```python
from build123d import *

# Parameters (mm, degrees)
SKETCH_1_R          = 1.5
EXTRUDE_1_DEPTH     = 3
SKETCH_2_R          = 1.5
EXTRUDE_4_DEPTH     = 6
FILLET_1_R          = 1
SKETCH_3_R          = 1.5
CUT_EXTRUDE_1_DEPTH = 10


with BuildPart() as part:
    # ｽｹｯﾁ1 → ﾎﾞｽ - 押し出し1 (new body)
    with BuildSketch(Plane.XY):
        with BuildLine():
            Line((-3, 0), (-3, -30))
            ThreePointArc((-3, -30), (0, -33), (3, -30))
            Line((3, -30), (3, 0))
            ThreePointArc((3, 0), (0, 3), (-3, 0))
        make_face()
        Circle(SKETCH_1_R, mode=Mode.SUBTRACT)
        with Locations(Location((0, -30, 0), (0, 0, 180))):
            Circle(SKETCH_1_R, mode=Mode.SUBTRACT)
    extrude(amount=EXTRUDE_1_DEPTH)

    # ｽｹｯﾁ2 → ﾎﾞｽ - 押し出し4 (add)
    with BuildSketch(Plane(origin=(3, 0, 0), x_dir=(0, 0, -1), z_dir=(1, 0, 0))):
        with BuildLine():
            Line((0, -14), (-5, -14))
            ThreePointArc((-5, -14), (-8, -17), (-5, -20))
            Line((-5, -20), (0, -20))
            Line((0, -20), (0, -14))
        make_face()
        with Locations(Location((-5, -17, 0), (0, 0, 90))):
            Circle(SKETCH_2_R, mode=Mode.SUBTRACT)
    extrude(amount=-EXTRUDE_4_DEPTH)

    # ﾌｨﾚｯﾄ1
    fillet_1_edges = [part.edges().sort_by_distance(p)[0] for p in [
        (0, -14, 3),
        (0, -20, 3),
    ]]
    fillet(fillet_1_edges, radius=FILLET_1_R)

    # ｽｹｯﾁ3 → ｶｯﾄ - 押し出し1 (cut)
    with BuildSketch(Plane(origin=(0, 0, 0), x_dir=(-1, 0, 0), z_dir=(0, 0, -1))):
        with Locations((0, -10)):
            Circle(SKETCH_3_R)
    extrude(amount=-CUT_EXTRUDE_1_DEPTH, mode=Mode.SUBTRACT)


solid = part.part
```
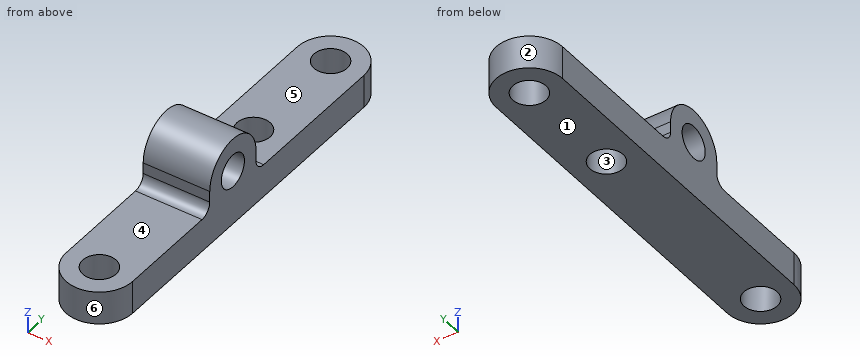
The model under review builds one solid part; all positions refer to its coordinate system, in mm. Face numbers are marked on the shaded views. A direction names the side the tool comes from. Give positions to 0.01 mm unless a question says otherwise; leave off trailing zeros. Order: outer loops, then holes, each group sorted by start corner. A loop starts at its lowest first (then second) coordinate and runs counter-clockwise, first axis right, second up. Notation, with made-up numbers: (87, 31.25) - (112, 31.25) arc R14 cw to (112, 47.25) - close; hole circle Ø4 at (70, 16). An arc over 180 degrees is marked (long way). Use CSV: the item, a comma, the result in double quotes. Start each with the question number.
Q1. We need section B-B, the plane y = -17. Write out the cut boundary in (x, z).
Q2. We need section A-A, the plane x = 0. Write out the cut boundary in (y, z), and give its area (3 significant figures).
Q3. The part is to be moulded in two halves that separate along X. For the marked faces 1, 2 and 3, say which applies: +X half, -X half, draft (parallel to the pull), parting line (faces both ways), or undercut.
Q4. To check wall thickness, follow line 1 along Y through (x, z) = (0, 0.9); line 2 along Y through (x, z) = (0.8, 0.75); line 3 along X through (y, z) = (-30, 1.4). State the ranges of each line that lie inside material, in increasing order. Write a range as [from, to].
Q5. Clearance check with flat-ended pins moving along their axes: pin 1 Ø3 at (x, y) = (-1, -30) entering from +Z; pin 2 Ø1.1 at (x, z) = (-1, 4.5) entering from +Y; pin 3 Ø3 at (x, z) = (-1, 6.5) entering from -Y; pin 4 Ø3.5 at (y, z) = (-17, 5) entering from +X. State where each tip first meets the part, or that it passes through.
Q6. We need section D-D, the plane x = -2.3. Write out the cut boundary in (y, z).
Q7. We need section C-C, the plane z = 6. Write out the cut boundary in (x, y), and give its area (3 significant figures).
Q8. Tool access review of the marked faces 4, 5 and 6: name each direction out of +Z, -Z, +X, -X, +Y, -Y from which nothing blocks a thin tool from reaching the whole face with its end or side.
Outcome:
1,outline,"(-3, 0) - (3, 0) - (3, 3.5) - (-3, 3.5) - close; (-3, 6.5) - (3, 6.5) - (3, 8) - (-3, 8) - close"
2,outline,"(-33, 0) - (-31.5, 0) - (-31.5, 3) - (-33, 3) - close; (-28.5, 0) - (-11.5, 0) - (-11.5, 3) - (-13, 3) arc R1 cw to (-14, 4) - (-14, 5) arc R3 ccw to (-20, 5) - (-20, 4) arc R1 cw to (-21, 3) - (-28.5, 3) - close; (-8.5, 0) - (-1.5, 0) - (-1.5, 3) - (-8.5, 3) - close; (1.5, 0) - (3, 0) - (3, 3) - (1.5, 3) - close; hole circle Ø3 at (-17, 5)"
2,area,"100 mm^2"
3,face 1,"draft"
3,face 2,"parting line"
3,face 3,"undercut"
4,line 1,"y = [-33, -31.5], [-28.5, -11.5], [-8.5, -1.5], [1.5, 3]"
4,line 2,"y = [-32.89, -31.27], [-28.73, -11.27], [-8.73, -1.27], [1.27, 2.89]"
4,line 3,"x = [-3, -1.5], [1.5, 3]"
5,pin 1,"stops at z = 3"
5,pin 2,"stops at y = -14"
5,pin 3,"stops at y = -20"
5,pin 4,"stops at x = 3"
6,outline,"(-31.93, 0) - (1.93, 0) - (1.93, 3) - (-13, 3) arc R1 cw to (-14, 4) - (-14, 5) arc R3 ccw to (-20, 5) - (-20, 4) arc R1 cw to (-21, 3) - (-31.93, 3) - close; hole circle Ø3 at (-17, 5)"
7,outline,"(-3, -19.83) - (3, -19.83) - (3, -18.12) - (-3, -18.12) - close; (-3, -15.88) - (3, -15.88) - (3, -14.17) - (-3, -14.17) - close"
7,area,"20.5 mm^2"
8,face 4,"+Z, +X, -X, -Y"
8,face 5,"+Z, +X, -X, +Y"
8,face 6,"+Z, -Z, -Y"
